Answer from the drawing. Dimensions are ordinates in mm from the lowest x, y and z of the part. Round coordinates to 2 decimals unless told otherwise and drop trailing zeros. Order: outer loops, then holes, each group sorted by start corner. A loop starts at its lowest first (then second) coordinate and runs counter-clockwise, first axis right, second up. Notation, with made-up numbers: M 72.5,41.25 L 122.5,41.25 A32 ccw 122.5,80.25 Z; hole C 9.25,-33.5 d9. An arc over 180 degrees is marked long. Answer as a JSON object with one key per item and string values. Group by question number.
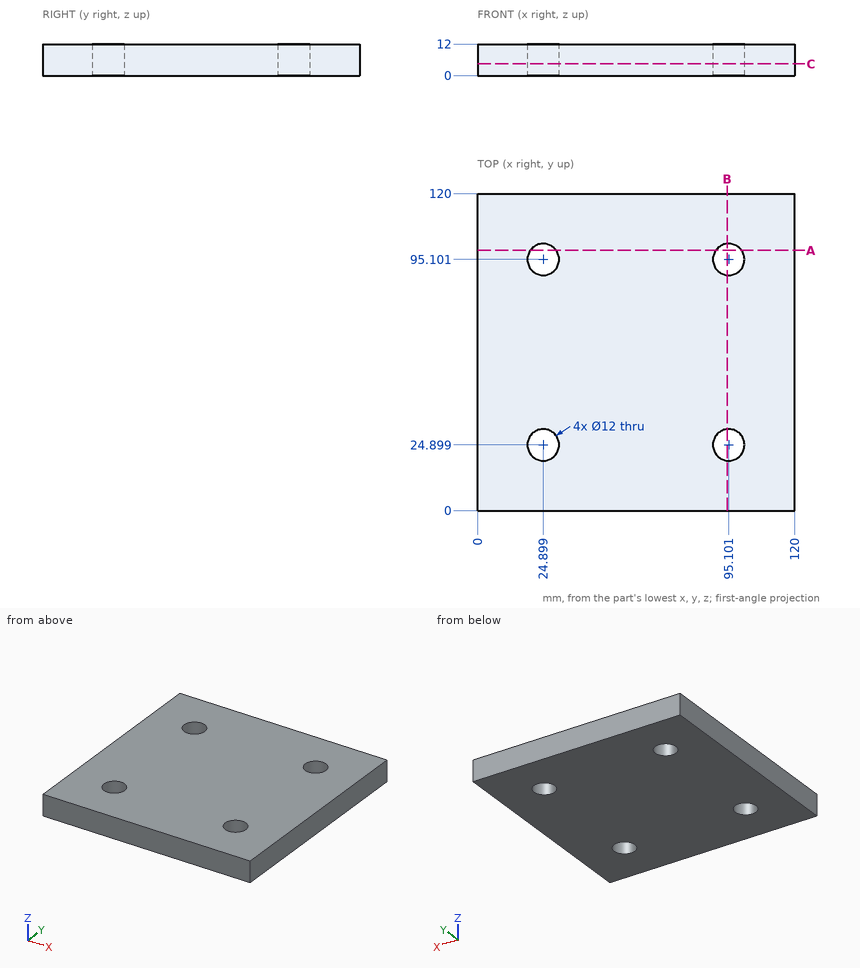
Item 1: Find section C-C (z = 4.5). Give the vertices of the cut face in (x, y), and give its area (3 significant figures).
Item 2: Find section B-B (x = 94.5). Give the vertices of the cut face in (y, z), and give its area (3 significant figures).
Item 3: Find section A-A (y = 98.5). Give the vertices of the cut face in (x, z) (1 decimal), and give its area (3 significant figures).
Item 4: Consider L1, parallel to Y at x = 91, z = 9.5; L2, parallel to Y at x = 93, z = 7.25; L3, parallel to X at y = 21, z = 6.5. Determine where each line is inside the solid, lowest interval first.
Responses:
{
 "1": {"outline": "M 0,0 L 120,0 L 120,120 L 0,120 Z; hole C 24.9,24.9 d12; hole C 24.9,95.1 d12; hole C 95.1,24.9 d12; hole C 95.1,95.1 d12", "area": "13,900 mm^2"},
 "2": {"outline": "M 0,0 L 18.93,0 L 18.93,12 L 0,12 Z; M 30.87,0 L 89.13,0 L 89.13,12 L 30.87,12 Z; M 101.07,0 L 120,0 L 120,12 L 101.07,12 Z", "area": "1,150 mm^2"},
 "3": {"outline": "M 0,0 L 20,0 L 20,12 L 0,12 Z; M 29.8,0 L 90.2,0 L 90.2,12 L 29.8,12 Z; M 100,0 L 120,0 L 120,12 L 100,12 Z", "area": "1,200 mm^2"},
 "4": {"L1": "y = 0 to 20.52, 29.28 to 90.72, 99.48 to 120", "L2": "y = 0 to 19.28, 30.52 to 89.48, 100.72 to 120", "L3": "x = 0 to 20.34, 29.46 to 90.54, 99.66 to 120"}
}
